The model under review builds one solid part; all positions refer to its coordinate system, in mm. A direction names the side the tool comes from. Round coordinates to 2 decimals unless told otherwise and drop trailing zeros. Write each loop counter-clockwise with the first axis right and the second up, starting at its lowest first coordinate (ties: lowest second). Pieces come first, ordered by that corner, then holes. Notation, with made-up numbers: (-34.5, 45.5) - (-13.5, 45.5) arc R7 cw to (-13.5, 49.5) - close; hole circle Ø3 at (-33, -4.75). An arc over 180 degrees is marked (long way). Use one line per item in the form item = value.
from build123d import *

# Parameters (mm, degrees)
F0_W      = 114.5
F0_H      = 52.4
F1_DEPTH  = 1.6
F2_R      = 0.6
F3_W      = 52.4
F3_H      = 3.2
F4_DEPTH  = 1
F5_R      = 0.6
F6_W      = 52.4
F6_H      = 3.2
F7_DEPTH  = 1
F8_R      = 0.6
F10_DEPTH = 1.6


with BuildPart() as f1:
    # F0 (on Top) → F1 (new body)
    with BuildSketch(Plane.XY):
        with Locations((57.25, 26.2)):
            Rectangle(F0_W, F0_H)
    extrude(amount=F1_DEPTH)

    # F2
    f2_edges = [f1.edges().sort_by_distance(p)[0] for p in [
        (57.25, 0, 1.6),
        (57.25, 52.4, 1.6),
    ]]
    fillet(f2_edges, radius=F2_R)

    # F3 (on face) → F4 (join)
    with BuildSketch(Plane.YZ.offset(114.5)):
        with Locations((26.2, 1.6)):
            Rectangle(F3_W, F3_H)
    extrude(amount=F4_DEPTH)

    # F5
    f5_edges = [f1.edges().sort_by_distance(p)[0] for p in [
        (115, 52.4, 3.2),
        (115, 0, 3.2),
    ]]
    fillet(f5_edges, radius=F5_R)

    # F6 (on face) → F7 (join)
    with BuildSketch(Plane(origin=(0, 0, 0), x_dir=(0, -1, 0), z_dir=(-1, 0, 0))):
        with Locations((-26.2, 1.6)):
            Rectangle(F6_W, F6_H)
    extrude(amount=F7_DEPTH)

    # F8
    f8_edges = [f1.edges().sort_by_distance(p)[0] for p in [
        (-0.5, 0, 3.2),
        (-0.5, 52.4, 3.2),
    ]]
    fillet(f8_edges, radius=F8_R)

    # F9 (on face) → F10 (join, through all)
    with BuildSketch(Plane.XY.offset(1.6)):
        Polygon((0, 26.7), (0, 25.7), (114.5, 25.7), (114.5, 26.2), (114.5, 26.7), align=None)
    extrude(amount=F10_DEPTH)


solid = f1.part
(1) Add section A-A on x = 50. Write out the cut boundary in (y, z).
Geometry results:
outline = (0, 0) - (52.4, 0) - (52.4, 1) arc R0.6 ccw to (51.8, 1.6) - (26.7, 1.6) - (26.7, 3.2) - (25.7, 3.2) - (25.7, 1.6) - (0.6, 1.6) arc R0.6 ccw to (0, 1) - close
(2) Insertion check: P1, Ø1.3, axis at x = 52.5, z = 2.5, coming from the +Y side; P2, Ø12.5, axis at x = 48, y = 41, coming from the +Z side; P3, Ø1.5, axis at x = 99, z = 2, coming from the +Y side. Each pin has a flat end and moves straight along its axis. Give the tip position at first contact, or say it passes through.
Geometry results:
P1 = 26.7
P2 = 1.6
P3 = 52.35
(3) Add section B-B on y = 31. Write out the cut boundary in (x, z).
Geometry results:
outline = (-1, 0) - (115.5, 0) - (115.5, 3.2) - (114.5, 3.2) - (114.5, 1.6) - (0, 1.6) - (0, 3.2) - (-1, 3.2) - close
(4) The part is to be moulded in two halves that separate along X. For faces 4 (the flat face through (0, 40, 2)), 5 (the flat face through (58, 27, 0)), 6 (the flat face through (115.5, 26, 2)), say which applies: +X half, -X half, draft (parallel to the pull), parting line (faces both ways), or undercut.
Geometry results:
face_4 = undercut
face_5 = draft
face_6 = +X half
(5) Machinability: for faces 1 (the flat face through (56, 13, 1.6)), 2 (the flat face through (-1, 27, 2)), 3 (the flat face through (56, 39, 1.6)), which of the approach directions +Z, -Z, +X, -X, +Y, -Y give a long, thin tool a straight path to every point of the face, cutting with its end or side? Answer none if there is none.
Geometry results:
face_1 = +Z, -Y
face_2 = +Z, -Z, -X, +Y, -Y
face_3 = +Z, +Y
(6) To check wall thickness, follow L1, parallel to X at y = 31, z = 2.2; L2, parallel to Z at x = 88.5, y = 21.5; L3, parallel to Y at x = 89, z = 1.9. State the ranges of each line that lie inside material, in increasing order.
Geometry results:
L1 = -1 to 0, 114.5 to 115.5
L2 = 0 to 1.6
L3 = 25.7 to 26.7
